Part model, mm, in its own coordinate system. A direction names the side the tool comes from. Give positions to 0.01 mm unless a question says otherwise; leave off trailing zeros. Order: outer loops, then holes, each group sorted by start corner. A loop starts at its lowest first (then second) coordinate and runs counter-clockwise, first axis right, second up. Notation, with made-up numbers: M 78,35 L 137,35 A15 cw 137,61 Z; hole C -32,-37.5 d8. An arc over 180 degrees is marked long. Answer as a JSON object with one key per item and string values.
from build123d import *

# Parameters (mm, degrees)
SKETCH_1_W                = 42.3
SKETCH_1_H                = 42.3
EXTRUDE_1_DEPTH           = 34
HOLE_WIZARD_3_0_3_1_D     = 3
HOLE_WIZARD_3_0_3_1_DEPTH = 5
CHAMFER_1_SIZE            = 3


with BuildPart() as part:
    # 草图1 → 凸台-拉伸1 (new body)
    with BuildSketch(Plane.XY.offset(29)):
        with Locations((80, 0)):
            Rectangle(SKETCH_1_W, SKETCH_1_H)
    extrude(amount=-EXTRUDE_1_DEPTH)

    # 草图2 → 旋转1 (revolve)
    with BuildSketch(Plane.XZ):
        Polygon((82.5, 53), (80, 53), (80, 29), (91, 29), (91, 31), (82.5, 31), align=None)
    revolve(axis=Axis((80, 0, 53), (0, 0, -1)))

    # Ø3.0 (3) 直径孔1
    with Locations(Plane.XY.offset(29)):
        with Locations((95.5, 15.5), (95.5, -15.5), (64.5, -15.5), (64.5, 15.5)):
            Hole(HOLE_WIZARD_3_0_3_1_D / 2, depth=HOLE_WIZARD_3_0_3_1_DEPTH)

    # 倒角1
    chamfer_1_edges = [part.edges().sort_by_distance(p)[0] for p in [
        (58.85, 21.15, 12),
        (101.15, 21.15, 12),
        (101.15, -21.15, 12),
        (58.85, -21.15, 12),
    ]]
    chamfer(chamfer_1_edges, length=CHAMFER_1_SIZE)


solid = part.part
1. Cut at A-A on x = 95.5. Give the cut face in (y, z).
Worked answers:
{"outline": "M -21.15,-5 L 21.15,-5 L 21.15,29 L 17,29 L 17,24 L 14,24 L 14,29 L -14,29 L -14,24 L -17,24 L -17,29 L -21.15,29 Z"}
2. Two-plate mould, pull along X, no slides. Class faces 1 (the flat face through (58.85, 0, 12)), 2 (the flat face through (80, -21.15, 12)), 3 (the flat face through (65, -15, 24)): +X half, -X half, draft (parallel to the pull), parting line (faces both ways), or undercut.
Worked answers:
{"face 1": "-X half", "face 2": "draft", "face 3": "undercut"}
3. Cut at B-B on z = 26.5. Give the cut face in (x, y), plus the area to 3 significant figures.
Worked answers:
{"outline": "M 58.85,-18.15 L 61.85,-21.15 L 98.15,-21.15 L 101.15,-18.15 L 101.15,18.15 L 98.15,21.15 L 61.85,21.15 L 58.85,18.15 Z; hole C 64.5,-15.5 d3; hole C 64.5,15.5 d3; hole C 95.5,-15.5 d3; hole C 95.5,15.5 d3", "area": "1,740 mm^2"}
4. Probe line 1 along Y through (x, z) = (95.5, 26.4); line 2 along X through (y, z) = (15, 27); line 3 along Z through (x, y) = (81, -8.5). List the from-to ranges inside material, lowest first.
Worked answers:
{"line 1": "y = -21.15 to -17, -14 to 14, 17 to 21.15", "line 2": "x = 58.85 to 63.09, 65.91 to 94.09, 96.91 to 101.15", "line 3": "z = -5 to 31"}
5. Cut at D-D on y = -4.5. Give the cut face in (x, z).
Worked answers:
{"outline": "M 58.85,-5 L 101.15,-5 L 101.15,29 L 90.04,29 L 90.04,31 L 69.96,31 L 69.96,29 L 58.85,29 Z"}
6. Pin check, flat tips, straight feed: P1, Ø1.5, axis at x = 72, y = 0, coming from the +Z side; P2, Ø8, axis at x = 71.5, y = -14.5, coming from the +Z side; P3, Ø2, axis at y = -2.5, z = 41.5, coming from the -X side. Stop position of each tip, or through.
Worked answers:
{"P1": "stops at z = 31", "P2": "stops at z = 29", "P3": "stops at x = 78"}
7. Cut at C-C on y = 0. Give the cut face in (x, z), plus the area to 3 significant figures.
Worked answers:
{"outline": "M 58.85,-5 L 101.15,-5 L 101.15,29 L 91,29 L 91,31 L 82.5,31 L 82.5,53 L 77.5,53 L 77.5,31 L 69,31 L 69,29 L 58.85,29 Z", "area": "1,590 mm^2"}
8. Which spindle directions (+Z, -Z, +X, -X, +Y, -Y) get a long thin tool onto all of the face, cutting with end or side? Do faces 4 (the flat face through (96, 16, 24)), 5 (the flat face through (80, 0, -5)). Say none if no direction does.
Worked answers:
{"face 4": "+Z", "face 5": "-Z, +X, -X, +Y, -Y"}
